Source: CAD feature listing. Evaluate the final solid. Frame: model axes, mm. Face numbers are marked on the shaded views. A direction names the side the tool comes from. Round coordinates to 2 decimals unless told otherwise and drop trailing zeros. Loops run counter-clockwise (first coordinate to the right, second up) from the corner with the lowest first, then second, coordinate; pieces in that order, holes last. Notation, with made-up numbers: M -11.5,30 L -5.5,30 A15 cw -5.5,36 Z; hole C 1,18 d3. An arc over 180 degrees is marked long. Answer as CSV lines item,"result". Start each with the question number.
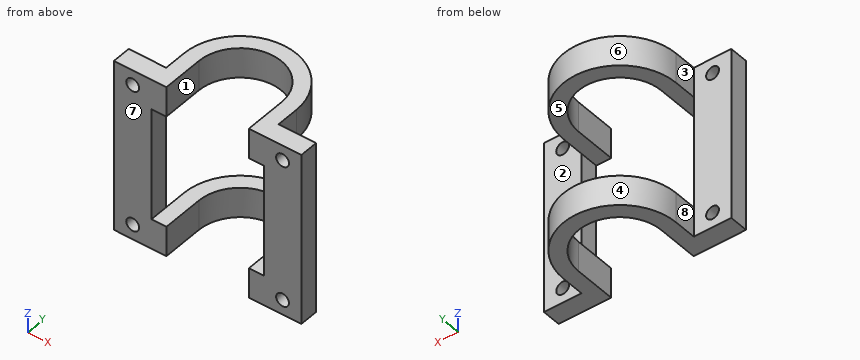
```python
from build123d import *

# Parameters (mm, degrees)
BOSS_EXTRUDE1_DEPTH = 10.16
SKETCH2_R           = 2.1828125
CUT_EXTRUDE1_DEPTH  = 7.62
SKETCH3_W           = 12.7
SKETCH3_H           = 19.05
BOSS_EXTRUDE2_DEPTH = 6.35


with BuildPart() as part:
    # Sketch1 → Boss-Extrude1 (new body)
    with BuildSketch(Plane.XY):
        with BuildLine():
            Line((0, 0), (0, 6.35))
            Line((0, 6.35), (12.7, 6.35))
            Line((12.7, 6.35), (12.7, 13.97))
            ThreePointArc((12.7, 13.97), (31.75, 33.02), (50.8, 13.97))
            Line((50.8, 13.97), (50.8, 6.35))
            Line((50.8, 6.35), (63.5, 6.35))
            Line((63.5, 6.35), (63.5, 0))
            Line((63.5, 0), (45.72, 0))
            Line((45.72, 0), (45.72, 13.97))
            ThreePointArc((45.72, 13.97), (31.75, 27.94), (17.78, 13.97))
            Line((17.78, 13.97), (17.78, 0))
            Line((17.78, 0), (0, 0))
        make_face()
    extrude(amount=BOSS_EXTRUDE1_DEPTH)

    # Sketch2 → Cut-Extrude1 (cut)
    with BuildSketch(Plane(origin=(0, 6.35, 0), x_dir=(1, 0, 0), z_dir=(0, 1, 0))):
        with Locations(Location((6.35, -5.08, 0), (0, 0, 270))):
            Circle(SKETCH2_R)
        with Locations(Location((57.15, -5.08, 0), (0, 0, 270))):
            Circle(SKETCH2_R)
    extrude(amount=-CUT_EXTRUDE1_DEPTH, mode=Mode.SUBTRACT)

    # Sketch3 → Boss-Extrude2 (add)
    with BuildSketch(Plane(origin=(0, 0, 0), x_dir=(1, 0, 0), z_dir=(0, 1, 0))):
        with Locations((6.35, -19.685)):
            Rectangle(SKETCH3_W, SKETCH3_H)
        with Locations((57.15, -19.685)):
            Rectangle(SKETCH3_W, SKETCH3_H)
    extrude(amount=BOSS_EXTRUDE2_DEPTH)

    # Mirror1: part across plane


with BuildPart() as part_1:
    add(part.part)
    add(part.part.mirror(Plane.XY.offset(29.21)))


solid = part_1.part
```
1) Section C-C, the plane y = 5.5. Return loops of the section in (x, z), and give its area (3 significant figures).
2) Ray query, line 1 along X through (y, z) = (12.5, 53.5); line 2 along Z through (x, y) = (6, 4); line 3 along Z through (x, y) = (34.5, 30). Return the intervals inside material, ascending.
3) Section A-A, the plane z = 5.08. Return loops of the section in (x, y), and give its area (3 significant figures).
4) Section D-D, the plane x = 25.5. Return loops of the section in (y, z).
5) Contact query for flat-ended pins moving along their axis: pin 1 Ø5 at (y, z) = (10, 7) entering from -X; pin 2 Ø5.5 at (x, z) = (6.35, 53.34) entering from +Y; pin 3 Ø4 at (x, z) = (57.15, 5.08) entering from -Y; pin 4 Ø1.5 at (y, z) = (8, 6.5) entering from +X. Output: stop coordinate, or through.
6) Access query for the marked faces 1, 2, 3 and 4. Directions: +Z, -Z, +X, -X, +Y, -Y. A direction counts if a zero-diameter tool reaches every point of the face in a straight line with its end or side. Return the directions, or none.
7) Section B-B, the plane x = 57.15. Return loops of the section in (y, z), and give its area (3 significant figures).
8) Mould query, pull axis X, two halves, no side actions, for the marked faces 5, 6, 7 and 8. Classes: pulls with the +X half, pulls with the -X half, needs draft (parallel to the pull), parting line crosses it, or undercut.
Findings below:
1,outline,"M 0,0 L 17.78,0 L 17.78,10.16 L 12.7,10.16 L 12.7,48.26 L 17.78,48.26 L 17.78,58.42 L 0,58.42 Z; M 45.72,0 L 63.5,0 L 63.5,58.42 L 45.72,58.42 L 45.72,48.26 L 50.8,48.26 L 50.8,10.16 L 45.72,10.16 Z; hole C 6.35,5.08 d4.37; hole C 6.35,53.34 d4.37; hole C 57.15,5.08 d4.37; hole C 57.15,53.34 d4.37"
1,area,"1,630 mm²"
2,line 1,"12.7 to 17.78, 45.72 to 50.8"
2,line 2,"0 to 2.93, 7.23 to 51.19, 55.49 to 58.42"
2,line 3,"0 to 10.16, 48.26 to 58.42"
3,outline,"M 0,0 L 4.17,0 L 4.17,6.35 L 0,6.35 Z; M 8.53,0 L 17.78,0 L 17.78,13.97 A13.97 cw 45.72,13.97 L 45.72,0 L 54.97,0 L 54.97,6.35 L 50.8,6.35 L 50.8,13.97 A19.05 ccw 12.7,13.97 L 12.7,6.35 L 8.53,6.35 Z; M 59.33,0 L 63.5,0 L 63.5,6.35 L 59.33,6.35 Z"
3,area,"511 mm²"
4,outline,"M 26.46,0 L 31.97,0 L 31.97,10.16 L 26.46,10.16 Z; M 26.46,48.26 L 31.97,48.26 L 31.97,58.42 L 26.46,58.42 Z"
5,pin 1,"x = 12.7"
5,pin 2,"y = 6.35"
5,pin 3,"through"
5,pin 4,"x = 50.8"
6,face 1,"+Z, -Z, -Y"
6,face 2,"+Z, -Z, +X, +Y"
6,face 3,"+Z, -Z, -X, +Y"
6,face 4,"+Z, -Z, +Y"
7,outline,"M 0,0 L 6.35,0 L 6.35,2.9 L 0,2.9 Z; M 0,7.26 L 6.35,7.26 L 6.35,51.16 L 0,51.16 Z; M 0,55.52 L 6.35,55.52 L 6.35,58.42 L 0,58.42 Z"
7,area,"316 mm²"
8,face 5,"undercut"
8,face 6,"parting line crosses it"
8,face 7,"needs draft"
8,face 8,"pulls with the -X half"
